Geometry: see drawing. Coordinates: mm, zero at the bounding-box minimum. A direction names the side the tool comes from. Round coordinates to 2 decimals unless told otherwise and drop trailing zeros. Order: outer loops, then holes, each group sorted by start corner. A loop starts at its lowest first (then second) coordinate and runs counter-clockwise, first axis right, second up. Notation, with made-up numbers: (-36.5, 35) -> (-5.5, 35) arc R15 cw to (-5.5, 44) -> close; hole circle Ø9 at (60, -21). An arc over 180 degrees is marked (long way). Write item = value, one per line. Start each with the question number.
(1) Cut plane B-B on y = 40. Return the cut outline in (x, z), then the cut area to 3 significant figures.
(2) Cut plane C-C on x = 30. Return the cut outline in (y, z).
(3) Ray query, line 1 (Z direction, x = 59.5, y = 18.5); line 2 (Y direction, x = 44, z = 74); line 3 (X direction, y = 29, z = 71) (3 decimals). Return the intervals inside material, ascending.
(4) Reachability of the marked faces 4 and 5 from +Z, -Z, +X, -X, +Y, -Y: full face, straight path, thin tool, end or side. Return the list, or none.
(5) Contact query for flat-ended pins moving along their axis: pin 1 Ø2 at (y, z) = (22, 82.5) entering from +X; pin 2 Ø1 at (x, z) = (101, 77) entering from +Y; pin 3 Ø1.8 at (x, z) = (31.5, 29.5) entering from -Y. Output: stop coordinate, or through.
(6) Cut plane A-A on z = 60. Return the cut outline in (x, y), then the cut area to 3 significant figures.
(7) Draft query along Z for the marked faces 1, 2 and 3. Return one class per face: released by +Z, released by -Z, zero draft, split by the parting line, or undercut.
(8) Cut plane D-D on z = 90. Return the cut outline in (x, y).
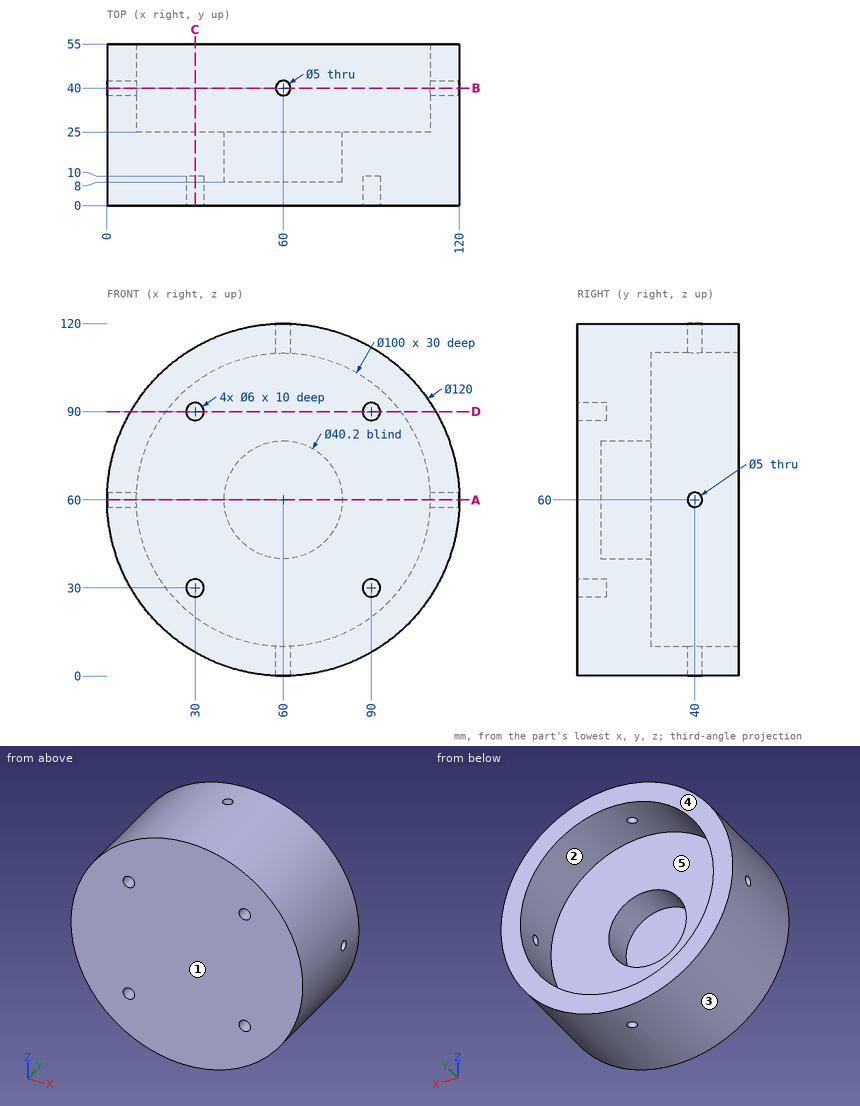
Evaluation:
q1.outline = (0.05, 57.5) arc R60 ccw to (57.5, 0.05) -> (57.5, 10.06) arc R50 cw to (10.06, 57.5) -> close; (0.05, 62.5) -> (10.06, 62.5) arc R50 cw to (57.5, 109.94) -> (57.5, 119.95) arc R60 ccw to start; (62.5, 0.05) arc R60 ccw to (119.95, 57.5) -> (109.94, 57.5) arc R50 cw to (62.5, 10.06) -> close; (62.5, 109.94) arc R50 cw to (109.94, 62.5) -> (119.95, 62.5) arc R60 ccw to (62.5, 119.95) -> close
q1.area = 3,260 mm^2
q2.outline = (0, 8.04) -> (55, 8.04) -> (55, 20) -> (25, 20) -> (25, 100) -> (55, 100) -> (55, 111.96) -> (0, 111.96) -> (0, 93) -> (10, 93) -> (10, 87) -> (0, 87) -> (0, 33) -> (10, 33) -> (10, 27) -> (0, 27) -> close
q3.line_1 = 0 to 39.91, 80.09 to 120
q3.line_2 = 0 to 25
q3.line_3 = 1.017 to 11.225, 108.775 to 118.983
q4.face_4 = +Z, -Z, +X, -X, +Y
q4.face_5 = +Y
q5.pin_1 = 116.02
q5.pin_2 = 25
q5.pin_3 = 10
q6.outline = (0, 0) -> (120, 0) -> (120, 37.5) -> (110, 37.5) -> (110, 25) -> (80.1, 25) -> (80.1, 8) -> (39.9, 8) -> (39.9, 25) -> (10, 25) -> (10, 37.5) -> (0, 37.5) -> close; (0, 42.5) -> (10, 42.5) -> (10, 55) -> (0, 55) -> close; (110, 42.5) -> (120, 42.5) -> (120, 55) -> (110, 55) -> close
q6.area = 2,820 mm^2
q7.face_1 = zero draft
q7.face_2 = undercut
q7.face_3 = split by the parting line
q8.outline = (8.04, 0) -> (27, 0) -> (27, 10) -> (33, 10) -> (33, 0) -> (87, 0) -> (87, 10) -> (93, 10) -> (93, 0) -> (111.96, 0) -> (111.96, 55) -> (100, 55) -> (100, 25) -> (20, 25) -> (20, 55) -> (8.04, 55) -> close
